from build123d import *

# Parameters (mm, degrees)
EXTRUDE_1_DEPTH           = 10
CUT_EXTRUDE_1_DEPTH       = 35.93431774
HOLE_WIZARD_M4_1_D        = 3.3
HOLE_WIZARD_M4_1_DEPTH    = 9.5
HOLE_WIZARD_M4_1_TIP      = 0.991420021
HOLE_WIZARD_2_D           = 3.2
HOLE_WIZARD_2_DEPTH       = 10
HOLE_WIZARD_2_CBORE_D     = 6
HOLE_WIZARD_2_CBORE_DEPTH = 3.4
HOLE_WIZARD_2_TIP         = 0.96137699
HOLE_WIZARD_M3_1_D        = 2.5


with BuildPart() as part:
    # 草图1 → 凸台-拉伸1 (new, symmetric)
    with BuildSketch(Plane(origin=(0, 0, 0), x_dir=(0, 0, -1), z_dir=(1, 0, 0))):
        Polygon((0, 0), (1.943803091, 10), (31.943803091, 10), (31.943803091, 0), align=None)
    extrude(amount=EXTRUDE_1_DEPTH, both=True)

    # 草图2 → 切除-拉伸1 (cut, through all)
    with BuildSketch(Plane(origin=(0, 10, 0), x_dir=(1, 0, 0), z_dir=(0, 1, 0))):
        with BuildLine():
            Line((-1, 31.943803091), (1, 31.943803091))
            Line((1, 31.943803091), (1, 24.881057025))
            ThreePointArc((1, 24.881057025), (0, 8.943803091), (-1, 24.881057025))
            Line((-1, 24.881057025), (-1, 31.943803091))
        make_face()
    extrude(amount=-CUT_EXTRUDE_1_DEPTH, mode=Mode.SUBTRACT)

    # M4 螺纹孔1
    with Locations(Plane(origin=(0, 0, 0), x_dir=(1, 0, 0), z_dir=(0, 0.19080899537654164, 0.9816271834476646))):
        with Locations((-6, 5.093583475), (6, 5.093583475)):
            Hole(HOLE_WIZARD_M4_1_D / 2, depth=HOLE_WIZARD_M4_1_DEPTH)
            with Locations((0, 0, -(HOLE_WIZARD_M4_1_DEPTH + HOLE_WIZARD_M4_1_TIP / 2))):  # 118° drill point
                Cone(0, HOLE_WIZARD_M4_1_D / 2, HOLE_WIZARD_M4_1_TIP, mode=Mode.SUBTRACT)

    # 打孔尺寸(%根据)内六角圆柱头螺钉的类型2
    with Locations(Plane(origin=(10, 0, 0), x_dir=(0, 0, -1), z_dir=(1, 0, 0))):
        with Locations((27.943803091, 5)):
            CounterBoreHole(HOLE_WIZARD_2_D / 2, HOLE_WIZARD_2_CBORE_D / 2, HOLE_WIZARD_2_CBORE_DEPTH, depth=HOLE_WIZARD_2_DEPTH)
            with Locations((0, 0, -(HOLE_WIZARD_2_DEPTH + HOLE_WIZARD_2_TIP / 2))):  # 118° drill point
                Cone(0, HOLE_WIZARD_2_D / 2, HOLE_WIZARD_2_TIP, mode=Mode.SUBTRACT)

    # M3 螺纹孔1 (through all)
    with Locations(Plane.ZY.offset(10)):
        with Locations((-27.943803091, 5)):
            Hole(HOLE_WIZARD_M3_1_D / 2)


solid = part.part
Verification items for the finished model (mm, model axes). A direction names the side the tool comes from. Coordinates: 2 decimals unless noted, no trailing zeros. Write each loop counter-clockwise with the first axis right and the second up, starting at its lowest first coordinate (ties: lowest second). Pieces come first, ordered by that corner, then holes. Notation, with made-up numbers: M 82.5,27.25 L 128.5,27.25 A29 cw 128.5,51.25 Z; hole C -37.75,-39 d9. An arc over 180 degrees is marked long. Use a Markdown table: item, result.
Q1. Set-up check for faces 1 (the face through (1, 6.18, -29.25)), 2 (the face through (10, 5, -16)), 3 (the face through (5, 10, -10)), 4 (the face through (6.3, 3.1, -11.1)), 5 (the face through (3.761, 5.07, -29.542)): record each of +Z, -Z, +X, -X, +Y, -Y from which the full face is reachable in a straight line by a thin tool's end or side.
Reply:
| item | result |
|---|---|
| face 1 | -Z, +Y, -Y |
| face 2 | +Z, -Z, +X, +Y, -Y |
| face 3 | +Z, -Z, +X, -X, +Y |
| face 4 | none |
| face 5 | +X |
Q2. Sectioned sample at D-D, the plane x = 0. Record the boundary of the cut face in (y, z), plus the area to 3 significant figures.
Reply:
| item | result |
|---|---|
| outline | M 0,-8.94 L 10,-8.94 L 10,-1.94 L 0,0 Z |
| area | 79.7 mm² |
Q3. Go/stop test with flat-tipped pins: P1, Ø3, axis at y = 4.5, z = -29, coming from the +X side; P2, Ø1, axis at x = 0, z = -27.5, coming from the -Y side; P3, Ø3, axis at x = -5.5, y = 2.5, coming from the +Z side; P4, Ø3, axis at y = 5, z = -27.94, coming from the -X side. Record where each tip stops, or that it passes through.
Reply:
| item | result |
|---|---|
| P1 | stops at x = 6.6 |
| P2 | passes through |
| P3 | stops at z = -0.19 |
| P4 | stops at x = -10 |
Q4. Sectioned sample at A-A, the plane x = -3. Record the boundary of the cut face in (y, z).
Reply:
| item | result |
|---|---|
| outline | M 0,-31.94 L 10,-31.94 L 10,-24.36 L 0,-24.36 Z; M 0,-9.53 L 10,-9.53 L 10,-1.94 L 0,0 Z; hole C 5,-27.94 d2.5 |
Q5. Sectioned sample at C-C, the plane z = -28.5. Record the boundary of the cut face in (x, y).
Reply:
| item | result |
|---|---|
| outline | M -10,0 L -1,0 L -1,3.88 L -10,3.88 Z; M -10,6.12 L -1,6.12 L -1,10 L -10,10 Z; M 1,0 L 10,0 L 10,2.05 L 6.6,2.05 L 6.6,3.5 L 1,3.5 Z; M 1,6.5 L 6.6,6.5 L 6.6,7.95 L 10,7.95 L 10,10 L 1,10 Z |
Q6. Sectioned sample at B-B, the plane z = -23. Record the boundary of the cut face in (x, y), plus the area to 3 significant figures.
Reply:
| item | result |
|---|---|
| outline | M -10,0 L -5.23,0 L -5.23,10 L -10,10 Z; M 5.23,0 L 10,0 L 10,10 L 5.23,10 Z |
| area | 95.5 mm² |
Q7. Thickness scan on line 1 (X direction, y = 9.25, z = -26); line 2 (X direction, y = 4.5, z = -15); line 3 (Z direction, x = -4.75, y = 9). Record the ranges inside material, lowest first.
Reply:
| item | result |
|---|---|
| line 1 | x = -10 to -1, 1 to 10 |
| line 2 | x = -10 to -7.76, 7.76 to 10 |
| line 3 | z = -31.94 to -23.38, -10.51 to -1.75 |
Q8. Draft check along Z on faces 6 (the face through (0.34, 5.07, -8.95)), 7 (the face through (-1, 6, -29)), 8 (the face through (-5, 5, -31.944)), 9 (the face through (0.14, 4.93, -0.96)). Enter one of: +Z half, -Z half, draft (parallel to the pull), parting line (faces both ways), or undercut.
Reply:
| item | result |
|---|---|
| face 6 | undercut |
| face 7 | draft |
| face 8 | -Z half |
| face 9 | +Z half |
